Verification items for the finished model (mm, model axes). A direction names the side the tool comes from. Give positions to 0.01 mm unless a question says otherwise; leave off trailing zeros. Write each loop counter-clockwise with the first axis right and the second up, starting at its lowest first coordinate (ties: lowest second). Pieces come first, ordered by that corner, then holes. Notation, with made-up numbers: (30, 82) -> (56, 82) arc R17 cw to (56, 100) -> close; hole circle Ø6 at (43, 66). An arc over 180 degrees is marked (long way). Answer as CSV lines item,"result". Start each with the question number.
1) Tool access check on faces 1 (the flat face through (-39.751, -86, -1)), 2 (the cylindrical face through (5.86, -48.097, 53.931)), 3 (the flat face through (-1, -76, -53.975)). Record the directions out of +Z, -Z, +X, -X, +Y, -Y that give a thin tool (end or side, any length) a straight path to the whole face; none if there is none.
2) Sectioned sample at A-A on y = -36.83. Record the cut outline in (x, z) (3 decimals), and give its area (3 significant figures).
3) Sectioned sample at D-D on y = -78. Record the cut outline in (x, z) (3 decimals), and give its area (3 significant figures).
4) Material ranges on L1, parallel to Z at x = -25, y = -29 (3 decimals); L2, parallel to X at y = -6, z = 68.5; L3, parallel to Z at x = 36.5, y = -78.5 (3 decimals), recorded low to high.
5) Sectioned sample at B-B on x = 32. Record the cut outline in (y, z) (3 decimals), and give its area (3 significant figures).
6) Sectioned sample at C-C on z = -8. Record the cut outline in (x, y).
7) Mould release check, pull along Z, two halves, no side actions. Record for faces 4 (the flat face through (1, -3, -76.2)), 5 (the flat face through (-1, -86, 50.8)), 6 (the flat face through (36.576, -3, -64)): released by +Z, released by -Z, zero draft, split by the parting line, or undercut.
8) Gauge pin test, flat ends, axial feed: pin 1 Ø2 at (x, y) = (25.5, -75) entering from +Z (3 decimals); pin 2 Ø20.5 at (x, z) = (-11, 69.5) entering from -Y; pin 3 Ø10 at (y, z) = (-53.5, 56) entering from -X. Record the tip position at first contact, or that the pin passes through.
```python
from build123d import *

# Parameters (mm, degrees)
F0_W      = 79.502
F0_H      = 101.6
F1_DEPTH  = 88.9
F2_W      = 85.852
F2_H      = 107.95
F3_DEPTH  = 25.4
F4_W      = 73.152
F4_H      = 95.25
F5_DEPTH  = 85.725
F6_W      = 73.152
F6_H      = 152.4
F7_DEPTH  = 6.35
F8_R      = 3.96875
F9_DEPTH  = 6.351
F10_W     = 79.502
F10_H     = 101.6
F10_W_2   = 73.152
F10_H_2   = 95.25
F11_DEPTH = 6.35
F12_R     = 12.7
F13_DEPTH = 6.35
F14_R     = 12.7
F15_DEPTH = 6.35


with BuildPart() as f1:
    # F0 (on Front) → F1 (new body)
    with BuildSketch(Plane.XZ):
        Rectangle(F0_W, F0_H)
    extrude(amount=F1_DEPTH)

    # F2 (on face) → F3 (join)
    with BuildSketch(Plane.XZ.offset(88.9)):
        Rectangle(F2_W, F2_H)
    extrude(amount=-F3_DEPTH)

    # F4 (on face) → F5 (cut)
    with BuildSketch(Plane.XZ.offset(88.9)):
        Rectangle(F4_W, F4_H)
    extrude(amount=-F5_DEPTH, mode=Mode.SUBTRACT)

    # F6 (on face) → F7 (join)
    with BuildSketch(Plane(origin=(0, 0, 0), x_dir=(-1, 0, 0), z_dir=(0, 1, 0))):
        Rectangle(F6_W, F6_H)
    extrude(amount=-F7_DEPTH)

    # F8 (on face) → F9 (cut, through all)
    with BuildSketch(Plane.XZ.offset(6.35)):
        with Locations((-19.8755, 67.437)):
            Circle(F8_R)
        with Locations((24.5745, 67.437)):
            Circle(F8_R)
        with Locations((-19.8755, -67.437)):
            Circle(F8_R)
        with Locations((24.5745, -67.437)):
            Circle(F8_R)
    extrude(amount=-F9_DEPTH, mode=Mode.SUBTRACT)

    # F10 (on face) → F11 (cut)
    with BuildSketch(Plane.XZ.offset(88.9)):
        Rectangle(F10_W, F10_H)
        Rectangle(F10_W_2, F10_H_2, mode=Mode.SUBTRACT)
    extrude(amount=-F11_DEPTH, mode=Mode.SUBTRACT)

    # F12 (on face) → F13 (join)
    with BuildSketch(Plane.XY.offset(50.8)):
        with Locations((0, -36.83)):
            Circle(F12_R)
    extrude(amount=F13_DEPTH)

    # F14 (on face) → F15 (join)
    with BuildSketch(Plane(origin=(0, 0, -50.8), x_dir=(1, 0, 0), z_dir=(0, 0, -1))):
        with Locations((0, 36.83)):
            Circle(F14_R)
    extrude(amount=F15_DEPTH)


solid = f1.part
```
Ans:
1,face 1,"-Y"
1,face 2,"+Z"
1,face 3,"-Z, +X, -X, -Y"
2,outline,"(-39.751, -50.8) -> (-12.7, -50.8) -> (-12.7, -57.15) -> (12.7, -57.15) -> (12.7, -50.8) -> (39.751, -50.8) -> (39.751, 50.8) -> (12.7, 50.8) -> (12.7, 57.15) -> (-12.7, 57.15) -> (-12.7, 50.8) -> (-39.751, 50.8) -> close; hole (-36.576, -47.625) -> (36.576, -47.625) -> (36.576, 47.625) -> (-36.576, 47.625) -> close"
2,area,"1,430 mm²"
3,outline,"(-42.926, -53.975) -> (42.926, -53.975) -> (42.926, 53.975) -> (-42.926, 53.975) -> close; hole (-36.576, -47.625) -> (36.576, -47.625) -> (36.576, 47.625) -> (-36.576, 47.625) -> close"
3,area,"2,300 mm²"
4,L1,"z = -50.8 to -47.625, 47.625 to 50.8"
4,L2,"x = -36.58 to -23.7, -16.05 to 20.75, 28.4 to 36.58"
4,L3,"z = -53.975 to -47.625, 47.625 to 53.975"
5,outline,"(-88.9, -53.975) -> (-63.5, -53.975) -> (-63.5, -50.8) -> (-6.35, -50.8) -> (-6.35, -76.2) -> (0, -76.2) -> (0, 76.2) -> (-6.35, 76.2) -> (-6.35, 50.8) -> (-63.5, 50.8) -> (-63.5, 53.975) -> (-88.9, 53.975) -> (-88.9, 50.8) -> (-82.55, 50.8) -> (-82.55, 47.625) -> (-6.35, 47.625) -> (-6.35, -47.625) -> (-82.55, -47.625) -> (-82.55, -50.8) -> (-88.9, -50.8) -> close"
5,area,"1,610 mm²"
6,outline,"(-42.93, -88.9) -> (-39.75, -88.9) -> (-39.75, -82.55) -> (-36.58, -82.55) -> (-36.58, -6.35) -> (36.58, -6.35) -> (36.58, -82.55) -> (39.75, -82.55) -> (39.75, -88.9) -> (42.93, -88.9) -> (42.93, -63.5) -> (39.75, -63.5) -> (39.75, 0) -> (-39.75, 0) -> (-39.75, -63.5) -> (-42.93, -63.5) -> close"
7,face 4,"released by -Z"
7,face 5,"undercut"
7,face 6,"zero draft"
8,pin 1,"stops at z = 53.975"
8,pin 2,"stops at y = -6.35"
8,pin 3,"stops at x = -5.01"
